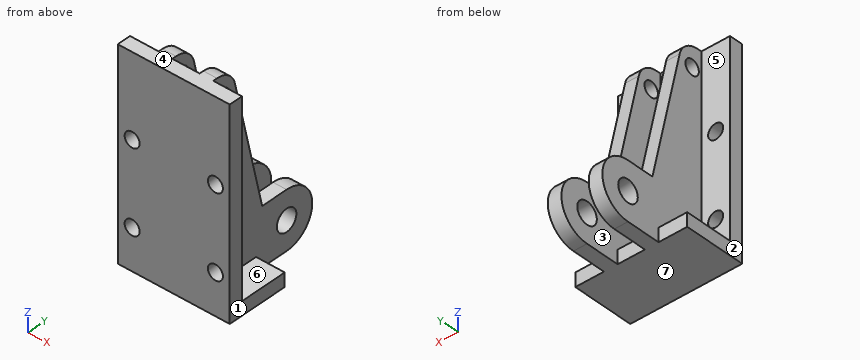
from build123d import *

# Parameters (mm, degrees)
BOSS_EXTRUDE1_DEPTH = 41
SKETCH2_R           = 8
SKETCH2_R_2         = 5.5
BOSS_EXTRUDE2_DEPTH = 10
SKETCH3_R           = 5.5
CUT_EXTRUDE1_DEPTH  = 10
FILLET1_R           = 15


with BuildPart() as part:
    # Sketch1 → Boss-Extrude1 (new, symmetric)
    with BuildSketch(Plane(origin=(0, 0, 0), x_dir=(0, 0, -1), z_dir=(1, 0, 0))):
        Polygon((0, 0), (-10, 0), (-10, -35), (-150, -35), (-150, -45), (0, -45), align=None)
    extrude(amount=BOSS_EXTRUDE1_DEPTH, both=True)

    # Sketch2 → Boss-Extrude2 (add)
    with BuildSketch(Plane(origin=(10, 0, 0), x_dir=(0, 0, -1), z_dir=(1, 0, 0))):
        with BuildLine():
            Line((-150, -35), (-150, -20))
            Line((-150, -20), (-42, 5))
            Line((-42, 5), (-42, 25))
            ThreePointArc((-42, 25), (-21, 46), (0, 25))
            Line((0, 25), (0, 0))
            Line((0, 0), (-10, 0))
            Line((-10, 0), (-10, -35))
            Line((-10, -35), (-150, -35))
        make_face()
        with Locations((-21, 25)):
            Circle(SKETCH2_R, mode=Mode.SUBTRACT)
        with Locations((-135, -27.5)):
            Circle(SKETCH2_R_2, mode=Mode.SUBTRACT)
    boss_extrude2 = extrude(amount=BOSS_EXTRUDE2_DEPTH)

    # Mirror1: Boss-Extrude2 across plane
    add(boss_extrude2.mirror(Plane(origin=(0, 0, 0), x_dir=(0, 0, 1), z_dir=(1, 0, 0))))

    # Sketch3 → Cut-Extrude1 (cut)
    with BuildSketch(Plane(origin=(0, -35, 0), x_dir=(1, 0, 0), z_dir=(0, 1, 0))):
        with Locations(Location((30.5, -30, 0), (0, 0, 270))):
            Circle(SKETCH3_R)
        with Locations(Location((30.5, -90, 0), (0, 0, 270))):
            Circle(SKETCH3_R)
        with Locations(Location((-30.5, -90, 0), (0, 0, 270))):
            Circle(SKETCH3_R)
        with Locations(Location((-30.5, -30, 0), (0, 0, 270))):
            Circle(SKETCH3_R)
    extrude(amount=-CUT_EXTRUDE1_DEPTH, mode=Mode.SUBTRACT)

    # Fillet1
    fillet1_edges = [part.edges().sort_by_distance(p)[0] for p in [
        (15, -20, 150),
        (-15, -20, 150),
    ]]
    fillet(fillet1_edges, radius=FILLET1_R)


solid = part.part
Source: CAD feature listing. Evaluate the final solid. Frame: model axes, mm. Face numbers are marked on the shaded views. A direction names the side the tool comes from. Coordinates: 2 decimals unless noted, no trailing zeros. Order: outer loops, then holes, each group sorted by start corner. A loop starts at its lowest first (then second) coordinate and runs counter-clockwise, first axis right, second up. Notation, with made-up numbers: M 86.5,-37.5 L 104.5,-37.5 A19 cw 104.5,-16.5 Z; hole C 72.25,73 d1. An arc over 180 degrees is marked long. Write each question's results on one line, items separated by ' | '. Start each with the question number.
1. Draft query along X for the marked faces 1, 2, 3 and 4. Return one class per face: +X half, -X half, draft (parallel to the pull), parting line (faces both ways), or undercut.
2. Section C-C, the plane z = 90. Return the cut outline in (x, y).
3. Reachability of the marked faces 5, 6 and 7 from +Z, -Z, +X, -X, +Y, -Y: full face, straight path, thin tool, end or side. Return the list, or none.
4. Section B-B, the plane y = -37. Return the cut outline in (x, z).
5. Section A-A, the plane x = -30.5. Return the cut outline in (y, z).
6. Section D-D, the plane y = -2. Return the cut outline in (x, z).
7. Material intervals for L1, parallel to Z at x = -30, y = -42; L2, parallel to X at y = -40, z = 30; L3, parallel to Y at x = -14.25, z = 21, sorted ascending.
8. Pin query (flat end, axial travel): pin 1 (22 mm diameter, centred on x = 4.5, y = -17.5, fed in from +Z); pin 2 (12 mm diameter, centred on x = -0.5, z = 47, fed in from +Y); pin 3 (12.5 mm diameter, centred on y = -27.5, z = 135, fed in from +X); pin 4 (12.5 mm diameter, centred on x = 30.5, z = 90, fed in from -Y). Return the tip coordinate at first contact, or that it passes through.
Solution:
1) face 1: +X half | face 2: -X half | face 3: undercut | face 4: draft
2) outline: M -41,-45 L -36,-45 L -36,-35 L -41,-35 Z; M -25,-45 L 25,-45 L 25,-35 L 20,-35 L 20,-6.11 L 10,-6.11 L 10,-35 L -10,-35 L -10,-6.11 L -20,-6.11 L -20,-35 L -25,-35 Z; M 36,-45 L 41,-45 L 41,-35 L 36,-35 Z
3) face 5: +Z, -X, +Y | face 6: +Z, +X, +Y | face 7: -Z, +X, -X, +Y, -Y
4) outline: M -41,0 L 41,0 L 41,150 L -41,150 Z; hole C -30.5,30 d11; hole C -30.5,90 d11; hole C 30.5,30 d11; hole C 30.5,90 d11
5) outline: M -45,0 L 0,0 L 0,10 L -35,10 L -35,24.5 L -45,24.5 Z; M -45,35.5 L -35,35.5 L -35,84.5 L -45,84.5 Z; M -45,95.5 L -35,95.5 L -35,150 L -45,150 Z
6) outline: M -41,0 L 41,0 L 41,10 L 20,10 L 20,72.24 L 10,72.24 L 10,10 L -10,10 L -10,72.24 L -20,72.24 L -20,10 L -41,10 Z
7) L1: 0 to 24.52, 35.48 to 84.52, 95.48 to 150 | L2: -41 to -36, -25 to 25, 36 to 41 | L3: -45 to 17, 33 to 46
8) pin 1: z = 149.18 | pin 2: y = -35 | pin 3: x = 20 | pin 4: y = -45
